```python
from build123d import *

# Parameters (mm, degrees)
SKETCH_1_W          = 20
SKETCH_1_H          = 5
SKETCH_1_R          = 0.8
EXTRUDE_1_DEPTH     = 2.2
SKETCH_2_W          = 20
SKETCH_2_H          = 6.2
EXTRUDE_2_DEPTH     = 3
SKETCH_3_W          = 5
SKETCH_3_H          = 5.5
EXTRUDE_3_DEPTH     = 20
SKETCH_4_W          = 4.5
SKETCH_4_H          = 5
CUT_EXTRUDE_1_DEPTH = 70.742831173
CUT_EXTRUDE_2_DEPTH = 5


with BuildPart() as part:
    # 草图1 → 凸台-拉伸1 (new body)
    with BuildSketch(Plane(origin=(0, 0, 0), x_dir=(1, 0, 0), z_dir=(0, 1, 0))):
        with Locations((10, -2.5)):
            Rectangle(SKETCH_1_W, SKETCH_1_H)
        with Locations(Location((4, -2.5, 0), (0, 0, 270))):
            Circle(SKETCH_1_R, mode=Mode.SUBTRACT)
        with Locations(Location((16, -2.5, 0), (0, 0, 270))):
            Circle(SKETCH_1_R, mode=Mode.SUBTRACT)
    extrude(amount=EXTRUDE_1_DEPTH)

    # 草图2 → 凸台-拉伸2 (add)
    with BuildSketch(Plane.XY.offset(5)):
        with Locations((10, 3.1)):
            Rectangle(SKETCH_2_W, SKETCH_2_H)
    extrude(amount=EXTRUDE_2_DEPTH)

    # 草图3 → 凸台-拉伸3 (add, through all)
    with BuildSketch(Plane(origin=(20, 0, 0), x_dir=(0, 0, -1), z_dir=(1, 0, 0))):
        Polygon((-58, -10.55), (-58, -16.05), (-8, 0), (-8, 6.2), align=None)
        with Locations((-60.5, -13.3)):
            Rectangle(SKETCH_3_W, SKETCH_3_H)
    extrude(amount=-EXTRUDE_3_DEPTH)

    # 草图4 → 切除-拉伸1 (cut, through all)
    with BuildSketch(Plane(origin=(0, 6.2, 0), x_dir=(1, 0, 0), z_dir=(0, 1, 0))):
        Polygon((4.5, -58), (0, -18), (0, -58), align=None)
        Polygon((20, -58), (20, -18), (15.5, -58), align=None)
        with Locations((17.75, -60.5)):
            Rectangle(SKETCH_4_W, SKETCH_4_H)
        with Locations((2.25, -60.5)):
            Rectangle(SKETCH_4_W, SKETCH_4_H)
    extrude(amount=-CUT_EXTRUDE_1_DEPTH, mode=Mode.SUBTRACT)

    # 草图5 → 切除-拉伸2 (cut)
    with BuildSketch(Plane.XY.offset(63)):
        with BuildLine():
            Line((15.5, -10.55), (4.5, -10.55))
            Line((4.5, -10.55), (4.5, -16.05))
            Line((4.5, -16.05), (7.6, -16.05))
            ThreePointArc((7.6, -16.05), (10, -13.65), (12.4, -16.05))
            Line((12.4, -16.05), (15.5, -16.05))
            Line((15.5, -16.05), (15.5, -10.55))
        make_face()
    extrude(amount=-CUT_EXTRUDE_2_DEPTH, mode=Mode.SUBTRACT)


solid = part.part
```
Read the model definition and answer for the solid it produces. Units are mm, in the model's axes. A direction names the side the tool comes from. Coordinates: 2 decimals unless noted, no trailing zeros. Write each loop counter-clockwise with the first axis right and the second up, starting at its lowest first coordinate (ties: lowest second). Pieces come first, ordered by that corner, then holes. Notation, with made-up numbers: (-33, -39.75) -> (5, -39.75) arc R14 ccw to (5, -34.75) -> close; hole circle Ø10 at (74.25, -37). An arc over 180 degrees is marked (long way). Return JSON: item names as keys, results as strings.
1. A tool of negligible diameter and unlimited length cuts with its end or side. For faces 1 (the face through (10, 2.2, 2)), 2 (the face through (0, 2, 11)), 3 (the face through (10, 0, 4)), 4 (the face through (10, -13, 58)), from which of +Z, -Z, +X, -X, +Y, -Y can it reach the whole face along a straight path? Write none if from no direction.
Found:
{"face 1": "-Z, +X, -X, +Y", "face 2": "+Z, -Z, -X, +Y, -Y", "face 3": "-Z, +X, -X, -Y", "face 4": "+Z, +Y"}
2. Find the intervals of material crossed by line 1 along X through (y, z) = (1.45, 2.5); line 2 along Y through (x, z) = (7.75, 16.5); line 3 along Y through (x, z) = (7.5, 30), in increasing order. Write a range as from..to.
Found:
{"line 1": "0..3.2, 4.8..15.2, 16.8..20", "line 2": "-2.73..3.35", "line 3": "-7.06..-1.17"}
3. Each of these flat-tipped pins is pushed along its axis until it touches: P1, Ø6, axis at x = 14, z = 23.5, coming from the -Y side; P2, Ø6, axis at x = 12, y = -14, coming from the +Z side; P3, Ø5.5, axis at x = 10, z = 2, coming from the +Y side; P4, Ø5, axis at x = 9.5, z = 15.5, coming from the -Y side. Where does it stop, or does it pass through?
Found:
{"P1": "y = -5.94", "P2": "z = 63", "P3": "y = 2.2", "P4": "y = -3.21"}
4. A cutting plane is placed at B-B (x = 10). Determine the outline of the cut face in (y, z).
Found:
{"outline": "(-16.05, 58) -> (0, 8) -> (0, 0) -> (2.2, 0) -> (2.2, 5) -> (6.2, 5) -> (6.2, 8) -> (-10.55, 58) -> (-13.65, 58) -> (-13.65, 63) -> (-16.05, 63) -> close"}
5. Determine the mould class of faces 5 (the face through (15.22, 1.08, 2.33)), 6 (the face through (2.26, -6.56, 38.09)), 7 (the face through (10, 4, 5)) for opening direction X: pulls with the +X half, pulls with the -X half, needs draft (parallel to the pull), parting line crosses it, or undercut.
Found:
{"face 5": "undercut", "face 6": "pulls with the -X half", "face 7": "needs draft"}
6. A cutting plane is placed at C-C (y = -14.5). Determine the outline of the cut face in (x, z), and give its area (3 significant figures).
Found:
{"outline": "(3.96, 53.17) -> (16.04, 53.17) -> (15.5, 58) -> (11.83, 58) -> (11.83, 63) -> (8.17, 63) -> (8.17, 58) -> (4.5, 58) -> close", "area": "74.1 mm2"}
7. A cutting plane is placed at A-A (z = 2.5). Determine the outline of the cut face in (x, y), and give its area (3 significant figures).
Found:
{"outline": "(0, 0) -> (3.2, 0) -> (3.2, 2.2) -> (0, 2.2) -> close; (4.8, 0) -> (15.2, 0) -> (15.2, 2.2) -> (4.8, 2.2) -> close; (16.8, 0) -> (20, 0) -> (20, 2.2) -> (16.8, 2.2) -> close", "area": "37.0 mm2"}
8. A cutting plane is placed at D-D (z = 34). Determine the outline of the cut face in (x, y).
Found:
{"outline": "(1.8, -8.35) -> (18.2, -8.35) -> (18.2, -2.51) -> (1.8, -2.51) -> close"}
